```python
from build123d import *

# Parameters (mm, degrees)
SKETCH_R     = 2
SKETCH_R_2   = 1.5
PAD_DEPTH    = 2
SKETCH001_R  = 1.5
POCKET_DEPTH = 2.001


with BuildPart() as part:
    # Sketch → Pad (new body)
    with BuildSketch(Plane.XY):
        with BuildLine():
            Line((-20, -37.931886), (-20, -56))
            ThreePointArc((-20, -56), (-18.535534, -59.535534), (-15, -61))
            Line((-15, -61), (15, -61))
            ThreePointArc((15, -61), (18.535534, -59.535534), (20, -56))
            Line((20, -37.931886), (20, -56))
            ThreePointArc((24.441165, -35.300719), (21.470865, -35.35085), (20, -37.931886))
            ThreePointArc((24.441165, -35.300719), (34.685487, -33.08265), (33.941125, -22.627417))
            ThreePointArc((33.941125, 22.627417), (24.568542, 0), (33.941125, -22.627417))
            ThreePointArc((33.941125, 22.627417), (34.685487, 33.08265), (24.441165, 35.300719))
            Line((24.441165, 35.300719), (20.385, 35.300719))
            ThreePointArc((20.385, 35.300719), (16.5, 37.153216), (12.615, 35.300719))
            Line((-12.615, 35.300719), (12.615, 35.300719))
            ThreePointArc((-12.615, 35.300719), (-16.5, 37.153216), (-20.385, 35.300719))
            Line((-24.441165, 35.300719), (-20.385, 35.300719))
            ThreePointArc((-24.441165, 35.300719), (-34.685487, 33.08265), (-33.941125, 22.627417))
            ThreePointArc((-33.941125, -22.627417), (-24.568542, 0), (-33.941125, 22.627417))
            ThreePointArc((-33.941125, -22.627417), (-34.685487, -33.08265), (-24.441165, -35.300719))
            ThreePointArc((-20, -37.931886), (-21.470865, -35.35085), (-24.441165, -35.300719))
        make_face()
        with Locations((28.284271, 28.284271)):
            Circle(SKETCH_R, mode=Mode.SUBTRACT)
        with Locations((28.284271, -28.284271)):
            Circle(SKETCH_R, mode=Mode.SUBTRACT)
        with Locations((-28.284271, -28.284271)):
            Circle(SKETCH_R, mode=Mode.SUBTRACT)
        with Locations((-28.284271, 28.284271)):
            Circle(SKETCH_R, mode=Mode.SUBTRACT)
        with Locations((15.25, 15.25)):
            Circle(SKETCH_R_2, mode=Mode.SUBTRACT)
        with Locations((-15.25, 15.25)):
            Circle(SKETCH_R_2, mode=Mode.SUBTRACT)
        with Locations((-15.25, -15.25)):
            Circle(SKETCH_R_2, mode=Mode.SUBTRACT)
        with Locations((15.25, -15.25)):
            Circle(SKETCH_R_2, mode=Mode.SUBTRACT)
        with BuildLine():
            ThreePointArc((-7, -36), (-10, -33), (-13, -36))
            Line((-13, -36), (-13, -52))
            ThreePointArc((-13, -52), (-10, -55), (-7, -52))
            Line((-7, -36), (-7, -52))
        make_face(mode=Mode.SUBTRACT)
        with BuildLine():
            ThreePointArc((13, -36), (10, -33), (7, -36))
            Line((7, -36), (7, -52))
            ThreePointArc((7, -52), (10, -55), (13, -52))
            Line((13, -36), (13, -52))
        make_face(mode=Mode.SUBTRACT)
        with BuildLine():
            Line((-8.75337, 19.734959), (-3.521702, 14.543988))
            ThreePointArc((-3.521702, 14.543988), (0, 13.0933), (3.521702, 14.543988))
            Line((3.521702, 14.543988), (8.75337, 19.734959))
            ThreePointArc((8.75337, 19.734959), (9.854793, 25.188666), (5.231669, 28.284271))
            Line((5.231669, 28.284271), (-5.231669, 28.284271))
            ThreePointArc((-5.231669, 28.284271), (-9.854793, 25.188666), (-8.75337, 19.734959))
        make_face(mode=Mode.SUBTRACT)
        with BuildLine():
            Line((3.521702, -14.543988), (8.75337, -19.734959))
            ThreePointArc((5.231669, -28.284271), (9.854793, -25.188666), (8.75337, -19.734959))
            Line((5.231669, -28.284271), (-5.231669, -28.284271))
            ThreePointArc((-8.75337, -19.734959), (-9.854793, -25.188666), (-5.231669, -28.284271))
            Line((-8.75337, -19.734959), (-3.521702, -14.543988))
            ThreePointArc((3.521702, -14.543988), (0, -13.0933), (-3.521702, -14.543988))
        make_face(mode=Mode.SUBTRACT)
    extrude(amount=PAD_DEPTH)

    # Sketch001 → Pocket (cut, through all)
    with BuildSketch(Plane.XY.offset(2)):
        with Locations((-16.5, 33.5)):
            Circle(SKETCH001_R)
        with Locations((16.5, 33.5)):
            Circle(SKETCH001_R)
        with Locations((16.5, -56)):
            Circle(SKETCH001_R)
        with Locations((-16.5, -56)):
            Circle(SKETCH001_R)
    extrude(amount=-POCKET_DEPTH, mode=Mode.SUBTRACT)


solid = part.part
```
Geometry check sheet. Reference: the model listing, model coordinates, mm. A direction names the side the tool comes from. Coordinates: 2 decimals unless noted, no trailing zeros. Order: outer loops, then holes, each group sorted by start corner. A loop starts at its lowest first (then second) coordinate and runs counter-clockwise, first axis right, second up.
Item 1: Section check B-B (x = -0.5). Enter the section's corners in (y, z), plus the area to 3 significant figures.
Item 2: Depth check by flat-ended pin: pin 1 (1.8 mm diameter, centred on x = -16.5, y = -56, fed in from -Z); pin 2 (1 mm diameter, centred on y = 21, z = 1, fed in from +X); pin 3 (1 mm diameter, centred on y = -48, z = 1, fed in from -X); pin 4 (0.6 mm diameter, centred on x = 22.5, z = 1, fed in from +Y). Enter the tip coordinate at first touch or a pass-through.
Item 3: Mould release check, pull along Y, two halves, no side actions. Record for faces 3 (the cylindrical face through (-21.434, -35.373, 0.986)), 4 (the flat face through (-22, 35.301, 1)), 5 (the cylindrical face through (-16.75, -15.18, 0.99)): released by +Y, released by -Y, zero draft, split by the parting line, or undercut.
Item 4: Tool access check on faces 1 (the cylindrical face through (-16.438, 37.153, 0.986)), 2 (the cylindrical face through (-10, -55, 1)). Record the directions out of +Z, -Z, +X, -X, +Y, -Y that give a thin tool (end or side, any length) a straight path to the whole face; none if there is none.
Item 5: Scan lines: line 1 along Y through (x, z) = (2.5, 1.3); line 2 along X through (y, z) = (-51, 0.8); line 3 along Y through (x, z) = (29, 1.9). Record each from-to range of solid material in increasing order.
Item 6: Section check D-D (z = 1.45). Count the separate pieces of the cut face and the enclosed holes in it, plus the area to 3 significant figures.
Item 7: Section check C-C (x = -28). Enter the section's corners in (y, z), plus the area to 3 significant figures.
Item 8: Section check A-A (y = 24.5). Enter the section's corners in (x, z).
Check sheet entries:
1. outline: (-61, 0) - (-28.28, 0) - (-28.28, 2) - (-61, 2) - close; (-13.12, 0) - (13.12, 0) - (13.12, 2) - (-13.12, 2) - close; (28.28, 0) - (35.3, 0) - (35.3, 2) - (28.28, 2) - close
1. area: 132 mm2
2. pin 1: passes through
2. pin 2: stops at x = 32.87
2. pin 3: stops at x = -20
2. pin 4: stops at y = 35.3
3. face 3: released by -Y
3. face 4: released by +Y
3. face 5: undercut
4. face 1: +Z, -Z, +Y
4. face 2: +Z, -Z
5. line 1: y = -61 to -28.28, -13.76 to 13.76, 28.28 to 35.3
5. line 2: x = -20 to -13, -7 to 7, 13 to 20
5. line 3: y = -36.25 to -30.15, -26.42 to -16.25, 16.25 to 26.42, 30.15 to 36.25
6. separate pieces: 1
6. enclosed holes: 16
6. area: 4,520 mm2
7. outline: (-36.28, 0) - (-30.26, 0) - (-30.26, 2) - (-36.28, 2) - close; (-26.3, 0) - (-14.42, 0) - (-14.42, 2) - (-26.3, 2) - close; (14.42, 0) - (26.3, 0) - (26.3, 2) - (14.42, 2) - close; (30.26, 0) - (36.28, 0) - (36.28, 2) - (30.26, 2) - close
7. area: 71.6 mm2
8. outline: (-35.33, 0) - (-10.08, 0) - (-10.08, 2) - (-35.33, 2) - close; (10.08, 0) - (35.33, 0) - (35.33, 2) - (10.08, 2) - close
